```python
from build123d import *

# Parameters (mm, degrees)
RESSALTO_EXTRUS_O1_DEPTH   = 225
CORTE_EXTRUS_O1_DEPTH      = 226.9977876
CORTE_EXTRUS_O1_DEPTH_BACK = 226.9977876
ESBO_O2_R                  = 4


with BuildPart() as part:
    # Esboço1 → Ressalto-extrusão1 (new, symmetric)
    with BuildSketch(Plane.XY):
        Polygon((-13, -4.05), (-15, -4.05), (-15, -15), (-4.05, -15), (-4.05, -13), (-7.5, -13), (-7.5, -11.627272727), (-4.172727273, -8.3), (4.172727273, -8.3), (7.5, -11.627272727), (7.5, -13), (4.05, -13), (4.05, -15), (15, -15), (15, -4.05), (13, -4.05), (13, -7.5), (11.627272727, -7.5), (8.3, -4.172727273), (8.3, 4.172727273), (11.627272727, 7.5), (13, 7.5), (13, 4.05), (15, 4.05), (15, 15), (4.05, 15), (4.05, 13), (7.5, 13), (7.5, 11.627272727), (4.172727273, 8.3), (-4.172727273, 8.3), (-7.5, 11.627272727), (-7.5, 13), (-4.05, 13), (-4.05, 15), (-15, 15), (-15, 4.05), (-13, 4.05), (-13, 7.5), (-11.627272727, 7.5), (-8.3, 4.172727273), (-8.3, -4.172727273), (-11.627272727, -7.5), (-13, -7.5), align=None)
        with BuildLine():
            Line((-7.239339828, -5.233387445), (-5.125358847, -3.119406464))
            ThreePointArc((-5.125358847, -3.119406464), (-5.566897716, -2.238224702), (-5.858217272, -1.296645823))
            Line((-5.858217272, -1.296645823), (-7.3, -0.859788435))
            Line((-7.3, -0.859788435), (-7.3, 0.859788435))
            Line((-7.3, 0.859788435), (-5.858217272, 1.296645823))
            ThreePointArc((-5.858217272, 1.296645823), (-5.566897716, 2.238224702), (-5.125358847, 3.119406464))
            Line((-5.125358847, 3.119406464), (-7.239339828, 5.233387445))
            Line((-7.239339828, 5.233387445), (-5.233387445, 7.239339828))
            Line((-5.233387445, 7.239339828), (-3.119406464, 5.125358847))
            ThreePointArc((-3.119406464, 5.125358847), (-2.238224702, 5.566897716), (-1.296645823, 5.858217272))
            Line((-1.296645823, 5.858217272), (-0.859788435, 7.3))
            Line((-0.859788435, 7.3), (0.859788435, 7.3))
            Line((0.859788435, 7.3), (1.296645823, 5.858217272))
            ThreePointArc((1.296645823, 5.858217272), (2.238224702, 5.566897716), (3.119406464, 5.125358847))
            Line((3.119406464, 5.125358847), (5.233387445, 7.239339828))
            Line((5.233387445, 7.239339828), (7.239339828, 5.233387445))
            Line((7.239339828, 5.233387445), (5.125358847, 3.119406464))
            ThreePointArc((5.125358847, 3.119406464), (5.566897716, 2.238224702), (5.858217272, 1.296645823))
            Line((5.858217272, 1.296645823), (7.3, 0.859788435))
            Line((7.3, 0.859788435), (7.3, -0.859788435))
            Line((7.3, -0.859788435), (5.858217272, -1.296645823))
            ThreePointArc((5.858217272, -1.296645823), (5.566897716, -2.238224702), (5.125358847, -3.119406464))
            Line((5.125358847, -3.119406464), (7.239339828, -5.233387445))
            Line((7.239339828, -5.233387445), (5.233387445, -7.239339828))
            Line((5.233387445, -7.239339828), (3.119406464, -5.125358847))
            ThreePointArc((3.119406464, -5.125358847), (2.238224702, -5.566897716), (1.296645823, -5.858217272))
            Line((1.296645823, -5.858217272), (0.859788435, -7.3))
            Line((0.859788435, -7.3), (-0.859788435, -7.3))
            Line((-0.859788435, -7.3), (-1.296645823, -5.858217272))
            ThreePointArc((-1.296645823, -5.858217272), (-2.238224702, -5.566897716), (-3.119406464, -5.125358847))
            Line((-3.119406464, -5.125358847), (-5.233387445, -7.239339828))
            Line((-5.233387445, -7.239339828), (-7.239339828, -5.233387445))
        make_face(mode=Mode.SUBTRACT)
        Polygon((-11.005952384, -9), (-13, -9), (-13, -13), (-9, -13), (-9, -11.005952384), (-6.294047616, -8.3), (-8.3, -6.294047616), align=None, mode=Mode.SUBTRACT)
        Polygon((9, -11.005952384), (9, -13), (13, -13), (13, -9), (11.005952384, -9), (8.3, -6.294047616), (6.294047616, -8.3), align=None, mode=Mode.SUBTRACT)
        Polygon((11.005952384, 9), (13, 9), (13, 13), (9, 13), (9, 11.005952384), (6.294047616, 8.3), (8.3, 6.294047616), align=None, mode=Mode.SUBTRACT)
        Polygon((-9, 11.005952384), (-9, 13), (-13, 13), (-13, 9), (-11.005952384, 9), (-8.3, 6.294047616), (-6.294047616, 8.3), align=None, mode=Mode.SUBTRACT)
    extrude(amount=RESSALTO_EXTRUS_O1_DEPTH, both=True)

    # Esboço2 → Corte-extrusão1 (cut, two sides: drawn at the far end of the back side and taken through both)
    with BuildSketch(Plane(origin=(0, 0, 0), x_dir=(1, 0, 0), z_dir=(0, 1, 0)).offset(-CORTE_EXTRUS_O1_DEPTH_BACK)):
        with Locations(Location((0, -15, 0), (0, 0, 282.412424309))):
            Circle(ESBO_O2_R)
        with Locations(Location((0, 15, 0), (0, 0, 282.412424309))):
            Circle(ESBO_O2_R)
    extrude(amount=CORTE_EXTRUS_O1_DEPTH + CORTE_EXTRUS_O1_DEPTH_BACK, mode=Mode.SUBTRACT)


solid = part.part
```
Geometry: final body of the model. Coordinates: model frame, mm. Round coordinates to 2 decimals unless told otherwise and drop trailing zeros. Use one line per item in the form item = value. Start each with the question number.
Q1. Mould query, pull axis Y, two halves, no side actions, for faces 1 (the face through (10, 15, 3)), 2 (the face through (15, -10, 3)), 3 (the face through (-8.3, 0, 3)), 4 (the face through (-10, -15, 3)). Classes: +Y half, -Y half, draft (parallel to the pull), parting line (faces both ways), or undercut.
Q2. Cut plane A-A (z = -160.5). Count the separate pieces of the cut face and the enclosed holes in it, and give its area (3 significant figures).
Q3. Material intervals for line 1 (Z direction, x = -1, y = 8); line 2 (Z direction, x = -1.25, y = 7.5); line 3 (X direction, y = -11.5, z = -163), sorted ascending. Write a range as [from, to].
Q4. Pin query (flat end, axial travel): pin 1 Ø0.5 at (y, z) = (0.5, 92.5) entering from -X; pin 2 Ø4 at (x, z) = (-4, -161.5) entering from -Y; pin 3 Ø0.9 at (x, z) = (0, -114.5) entering from -Y. Return the tip coordinate at first contact, or that it passes through.
Geometry results:
q1.face_1 = +Y half
q1.face_2 = draft
q1.face_3 = undercut
q1.face_4 = -Y half
q2.separate_pieces = 1
q2.enclosed_holes = 5
q2.area = 341 mm^2
q3.line_1 = [-225, -18.87], [-11.13, 11.13], [18.87, 225]
q3.line_2 = [-225, -18.8], [-11.2, 11.2], [18.8, 225]
q3.line_3 = [-15, -13], [-9, -7.37], [7.37, 9], [13, 15]
q4.pin_1 = -8.3
q4.pin_2 = -15
q4.pin_3 = -8.3
